from build123d import *

# Parameters (mm, degrees)
CUT_EXTRUDE1_REACH      = 335.707
CUT_EXTRUDE1_END_RADIUS = 25
SKETCH2_R               = 1.5
CIRPATTERN1_COUNT       = 2


with BuildPart() as part:
    # Sketch1 → Revolve1 (revolve)
    with BuildSketch(Plane(origin=(0, 0, 0), x_dir=(0, 0, -1), z_dir=(1, 0, 0))):
        Polygon((0, 0), (-37.5, 0), (-37.5, 9), (-28, 9), (-28, 155.5), (-37.5, 155.5), (-37.5, 164.5), (-28, 164.5), (-28, 318), (-37.5, 318), (-37.5, 323), (-25, 323), (-25, 3), (0, 3), align=None)
    revolve(axis=Axis((0, 3, 0), (0, -1, 0)))

    # Cut-Extrude1: up to this cylinder (the profile starts outside it)
    cut_extrude1_end = Plane(origin=(0, 160, 0), z_dir=(0, 1, 0)) * Cylinder(CUT_EXTRUDE1_END_RADIUS, 722.414, mode=Mode.PRIVATE)
    # Sketch2 → Cut-Extrude1 (cut, up to the surface)
    with BuildSketch(Plane(origin=(0, 0, -37.5), x_dir=(-1, 0, 0), z_dir=(0, 0, -1)), mode=Mode.PRIVATE) as cut_extrude1_sk1:
        with Locations(Location((0, 160, 0), (0, 0, 90))):
            Circle(SKETCH2_R)
    cut_extrude1_tool1 = extrude(cut_extrude1_sk1.sketch, amount=-CUT_EXTRUDE1_REACH, mode=Mode.PRIVATE) - cut_extrude1_end
    cut_extrude1 = cut_extrude1_tool1.solids().sort_by_distance((0, 160, -37.5))[0]
    add(cut_extrude1, mode=Mode.SUBTRACT)

    # CirPattern1: Cut-Extrude1 ×2 about axis
    cirpattern1_axis = Axis((0, 3, 0), (0, 1, 0))
    for i in range(1, CIRPATTERN1_COUNT):
        add(cut_extrude1.rotate(cirpattern1_axis, i * 360 / CIRPATTERN1_COUNT), mode=Mode.SUBTRACT)


solid = part.part
Geometry check sheet. Reference: the model listing, model coordinates, mm. A direction names the side the tool comes from. Give positions to 0.01 mm unless a question says otherwise; leave off trailing zeros. Order: outer loops, then holes, each group sorted by start corner. A loop starts at its lowest first (then second) coordinate and runs counter-clockwise, first axis right, second up. Notation, with made-up numbers: (-36.75, -40) - (-17.75, -40) arc R21 cw to (-17.75, -4) - close; hole circle Ø3 at (76.5, -0.5). An arc over 180 degrees is marked (long way). Answer as a JSON object with one key per item and string values.
(1) Cross-section at C-C (x = -19.5). Record the cut outline in (y, z).
Report:
{"outline": "(0, -32.03) - (9, -32.03) - (9, -20.09) - (155.5, -20.09) - (155.5, -32.03) - (164.5, -32.03) - (164.5, -20.09) - (318, -20.09) - (318, -32.03) - (323, -32.03) - (323, -15.64) - (3, -15.64) - (3, 15.64) - (323, 15.64) - (323, 32.03) - (318, 32.03) - (318, 20.09) - (164.5, 20.09) - (164.5, 32.03) - (155.5, 32.03) - (155.5, 20.09) - (9, 20.09) - (9, 32.03) - (0, 32.03) - close"}
(2) Tool access check on faces 5 (the cylindrical face through (-37.18, 320.54, -4.88)), 6 (the flat face through (3, 9, -28)). Record the directions out of +Z, -Z, +X, -X, +Y, -Y that give a thin tool (end or side, any length) a straight path to the whole face; none if there is none.
Report:
{"face 5": "+Y, -Y", "face 6": "none"}
(3) Cross-section at A-A (y = 270). Record the cut outline in (x, z).
Report:
{"outline": "circle Ø56 at (0, 0); hole circle Ø50 at (0, 0)"}
(4) Cross-section at B-B (z = 0). Record the cut outline in (x, y).
Report:
{"outline": "(-37.5, 0) - (37.5, 0) - (37.5, 9) - (28, 9) - (28, 155.5) - (37.5, 155.5) - (37.5, 164.5) - (28, 164.5) - (28, 318) - (37.5, 318) - (37.5, 323) - (25, 323) - (25, 3) - (-25, 3) - (-25, 323) - (-37.5, 323) - (-37.5, 318) - (-28, 318) - (-28, 164.5) - (-37.5, 164.5) - (-37.5, 155.5) - (-28, 155.5) - (-28, 9) - (-37.5, 9) - close"}
(5) Material ranges on line 1 (Y direction, x = -19.5, z = 21.5); line 2 (Y direction, x = 0, z = 30); line 3 (Z direction, x = 0, y = 70), recorded low to high.
Report:
{"line 1": "0 to 9, 155.5 to 164.5, 318 to 323", "line 2": "0 to 9, 155.5 to 158.5, 161.5 to 164.5, 318 to 323", "line 3": "-28 to -25, 25 to 28"}
(6) Depth check by flat-ended pin: pin 1 Ø4 at (x, y) = (-2, 51) entering from -Z; pin 2 Ø2 at (y, z) = (108.5, 13.5) entering from -X; pin 3 Ø8 at (x, y) = (19, 170.5) entering from -Z. Enter the tip coordinate at first touch or a pass-through.
Report:
{"pin 1": "z = -28", "pin 2": "x = -25.05", "pin 3": "z = -23.64"}
(7) Draft check along Y on faces 1 (the cylindrical face through (10.724, 83.276, 25.865)), 2 (the flat face through (0, 3, 0)), 3 (the cylindrical face through (9.58, 160.76, 23.09)), 4 (the flat face through (-1, 0, 1)). Enter one of: released by +Y, released by -Y, zero draft, split by the parting line, or undercut.
Report:
{"face 1": "undercut", "face 2": "released by +Y", "face 3": "zero draft", "face 4": "released by -Y"}
